The model under review builds one solid part; all positions refer to its coordinate system, in mm. Give positions to 0.01 mm unless a question says otherwise; leave off trailing zeros. Order: outer loops, then holes, each group sorted by start corner. A loop starts at its lowest first (then second) coordinate and runs counter-clockwise, first axis right, second up. Notation, with made-up numbers: M -1,48.25 L 32,48.25 A11 ccw 32,52.25 Z; hole C -38.75,32 d10. An arc over 180 degrees is marked long. One line per question, with ' | ' between items. Start each with the question number.
1. We need section B-B on x = 46. Write out the cut boundary in (y, z), then the cut area to 3 significant figures.
2. Wall thickness on L1, parallel to Y at x = -46, z = 0.65; L2, parallel to Y at x = 46, z = 1.05; L3, parallel to Y at x = -25, z = 2.6: over which ranges is each line inside the solid? List them lowest first.
3. Insertion check: P1, Ø0.9, axis at y = -23.5, z = 1, coming from the -X side; P2, Ø5.5, axis at x = -46, y = -31, coming from the +Z side; P3, Ø1, axis at y = -3.5, z = 1, coming from the -X side. Each pin has a flat end and moves straight along its axis. Give the tip position at first contact, or say it passes through.
4. We need section A-A on x = 29. Write out the cut boundary in (y, z).
5. We need section D-D on y = 22.5. Write out the cut boundary in (x, z).
6. We need section C-C on z = 1.3. Count the separate pieces of the cut face and the enclosed holes in it, then the cut area to 3 significant figures.
```python
from build123d import *

# Parameters (mm, degrees)
F0_W     = 100
F0_H     = 70
F1_DEPTH = 4
F2_R     = 1.65
F3_DEPTH = 4
F2_W     = 17
F2_H     = 36
F2_W_2   = 59.3
F2_H_2   = 3
F4_DEPTH = 4
F6_DEPTH = 3
F7_R     = 3
F8_DEPTH = 2
F9_R     = 2


with BuildPart() as f1:
    # F0 (on Top) → F1 (new body)
    with BuildSketch(Plane.XY):
        Rectangle(F0_W, F0_H)
    extrude(amount=F1_DEPTH)

    # F2 (on face) → F3 (cut, through all)
    with BuildSketch(Plane.XY.offset(4)):
        with Locations((-46, 31)):
            Circle(F2_R)
        with Locations((46, 31)):
            Circle(F2_R)
        with Locations((46, -31)):
            Circle(F2_R)
        with Locations((-46, -31)):
            Circle(F2_R)
    extrude(amount=-F3_DEPTH, mode=Mode.SUBTRACT)

    # F2 (on face) → F4 (cut, through all)
    with BuildSketch(Plane.XY.offset(4)):
        with Locations((-34.15, -8.25)):
            Rectangle(F2_W, F2_H)
        Polygon((-42.65, -26.25), (-42.65, 9.75), (-42.65, 26.25), (-50, 26.25), (-50, -26.25), align=None)
        with Locations((13, 26.75)):
            Rectangle(F2_W_2, F2_H_2)
        Polygon((42.65, 25.25), (-16.65, 25.25), (-16.65, -21.25), (-15, -21.25), (35, -21.25), (42.65, -21.25), (48, -21.25), (48, 25.25), align=None)
    extrude(amount=-F4_DEPTH, mode=Mode.SUBTRACT)

    # F5 (on face) → F6 (cut)
    with BuildSketch(Plane.XY):
        Polygon((-50, -26.25), (-22.65, -26.25), (-22.65, -28.25), (-15, -28.25), (-15, -21.25), (35, -21.25), (35, -28.25), (42.65, -28.25), (42.65, -21.25), (48, -21.25), (48, 25.25), (42.65, 25.25), (42.65, 28.25), (-22.65, 28.25), (-22.65, 26.25), (-50, 26.25), align=None)
    extrude(amount=F6_DEPTH, mode=Mode.SUBTRACT)

    # F7 (on face) → F8 (cut)
    with BuildSketch(Plane.XY.offset(4)):
        with Locations((-46, 31)):
            Circle(F7_R)
        with Locations((46, 31)):
            Circle(F7_R)
        with Locations((46, -31)):
            Circle(F7_R)
        with Locations((-46, -31)):
            Circle(F7_R)
    extrude(amount=-F8_DEPTH, mode=Mode.SUBTRACT)

    # F9
    f9_edges = [f1.edges().sort_by_distance(p)[0] for p in [
        (-50, 35, 2),
        (-50, -35, 2),
        (50, -35, 2),
        (50, 35, 2),
        (-16.65, -21.25, 3.5),
        (-16.65, 28.25, 3.5),
        (-50, 26.25, 2),
        (-50, -26.25, 2),
        (-42.65, 26.25, 3.5),
        (-42.65, 9.75, 3.5),
        (-25.65, 9.75, 3.5),
        (-25.65, -26.25, 3.5),
    ]]
    fillet(f9_edges, radius=F9_R)


solid = f1.part
```
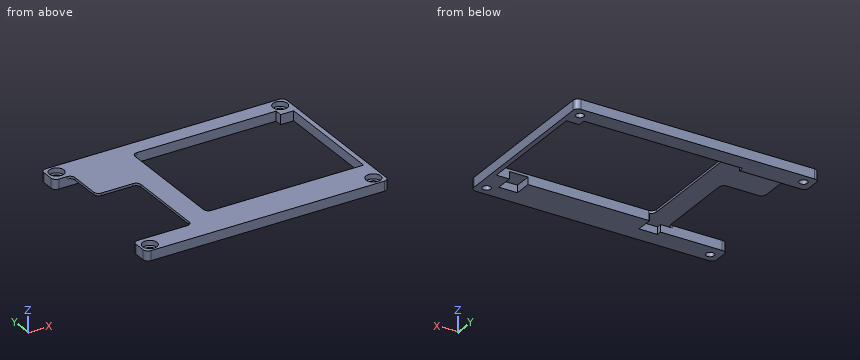
Entries:
1) outline: M -35,0 L -32.65,0 L -32.65,2 L -34,2 L -34,4 L -35,4 Z; M -29.35,0 L -21.25,0 L -21.25,4 L -28,4 L -28,2 L -29.35,2 Z; M 25.25,0 L 29.35,0 L 29.35,2 L 28,2 L 28,4 L 25.25,4 Z; M 32.65,0 L 35,0 L 35,4 L 34,4 L 34,2 L 32.65,2 Z | area: 56.8 mm^2
2) L1: y = -35 to -32.65, -29.35 to -26.25, 26.25 to 29.35, 32.65 to 35 | L2: y = -35 to -32.65, -29.35 to -21.25, 25.25 to 29.35, 32.65 to 35 | L3: y = -35 to -26.25, 26.25 to 35
3) P1: stops at x = -15 | P2: stops at z = 2 | P3: stops at x = 48
4) outline: M -35,0 L -21.25,0 L -21.25,4 L -35,4 Z; M 28.25,0 L 35,0 L 35,4 L 28.25,4 Z
5) outline: M -42.65,3 L -16.65,3 L -16.65,4 L -42.65,4 Z; M 48,0 L 50,0 L 50,4 L 48,4 Z
6) separate pieces: 1 | enclosed holes: 4 | area: 1,940 mm^2
